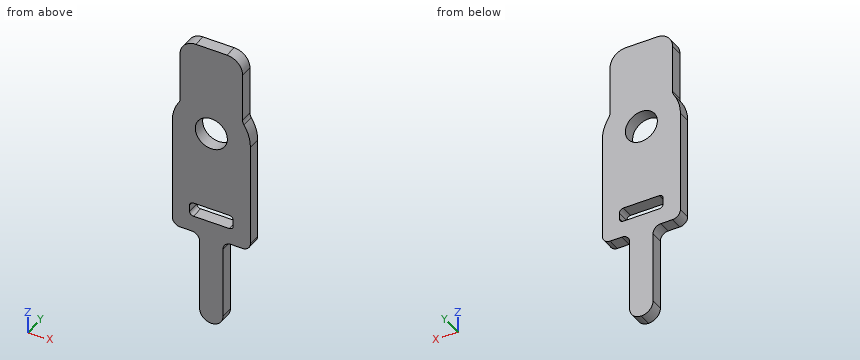
```python
from build123d import *

# Parameters (mm, degrees)
EXTRUDE_1_DEPTH = 1.6
FILLET_1_R      = 2
FILLET_2_R      = 1.5
FILLET_3_R      = 1
FILLET_4_R      = 0.5


with BuildPart() as part:
    # 草图1 → 凸台-拉伸1 (new body)
    with BuildSketch(Plane(origin=(0, 0, 0), x_dir=(1, 0, 0), z_dir=(0, 1, 0))):
        with BuildLine():
            Line((0, 37.4), (1.5, 37.4))
            Line((1.5, 37.4), (1.5, 25.7))
            Line((1.5, 25.7), (5, 25.7))
            Line((5, 25.7), (5, 11.5))
            ThreePointArc((5, 11.5), (4.74341649, 9.91886117), (4, 8.5))
            Line((4, 8.5), (4, 0))
            Line((4, 0), (0, 0))
            Line((0, 0), (0, 9.45))
            ThreePointArc((0, 9.45), (2.05, 11.5), (0, 13.55))
            Line((0, 13.55), (0, 21.8))
            Line((0, 21.8), (2.8, 21.8))
            Line((2.8, 21.8), (2.8, 23.6))
            Line((2.8, 23.6), (0, 23.6))
            Line((0, 23.6), (0, 37.4))
        make_face()
    extrude(amount=EXTRUDE_1_DEPTH)

    # 圆角1
    fillet_1_edges = [part.edges().sort_by_distance(p)[0] for p in [
        (4, 0.8, 0),
    ]]
    fillet(fillet_1_edges, radius=FILLET_1_R)

    # 圆角2
    fillet_2_edges = [part.edges().sort_by_distance(p)[0] for p in [
        (1.5, 0.8, -37.4),
    ]]
    fillet(fillet_2_edges, radius=FILLET_2_R - 0.0001)  # a hair under: the kernel refuses the full size

    # 圆角3
    fillet_3_edges = [part.edges().sort_by_distance(p)[0] for p in [
        (1.5, 0.8, -25.7),
        (5, 0.8, -25.7),
        (4, 0.8, -8.5),
    ]]
    fillet(fillet_3_edges, radius=FILLET_3_R)

    # 圆角4
    fillet_4_edges = [part.edges().sort_by_distance(p)[0] for p in [
        (2.8, 0.8, -21.8),
        (2.8, 0.8, -23.6),
    ]]
    fillet(fillet_4_edges, radius=FILLET_4_R)

    # 镜向1: part across plane


with BuildPart() as part_1:
    add(part.part)
    add(part.part.mirror(Plane(origin=(0, 1.6, -37.4), x_dir=(0, 0, 1), z_dir=(1, 0, 0))))


solid = part_1.part
```
The listing builds one solid part. Answer for the finished solid, in the listing's coordinates (mm). Give positions to 0.01 mm unless a question says otherwise; leave off trailing zeros. Order: outer loops, then holes, each group sorted by start corner. A loop starts at its lowest first (then second) coordinate and runs counter-clockwise, first axis right, second up. Notation, with made-up numbers: (30, 16.5) -> (42, 16.5) arc R10 cw to (42, 26.5) -> close; hole circle Ø8 at (12.25, 1). An arc over 180 degrees is marked (long way). Answer as CSV lines item,"result". Start each with the question number.
Q1. Find the intervals of material crossed by L1, parallel to Z at x = -0.75, y = 1.2; L2, parallel to X at y = 0.5, z = -11.5; L3, parallel to X at y = 0.9, z = -22.5, in increasing order.
Q2. Given pin 1 (0.5 mm diameter, centred on y = 1, z = -5, fed in from -X); pin 2 (2 mm diameter, centred on x = -0.5, z = -19.5, fed in from -Y); pin 3 (0.8 mm diameter, centred on y = 1, z = -30.5, fed in from +X), each flat-ended and moving along its own axis, determine where each tip first touches the part or whether it passes through.
Q3. A cutting plane is placed at A-A (y = 0.55). Count the separate pieces of the cut face and the enclosed holes in it, then the cut area to 3 significant figures.
Q4. A cutting plane is placed at D-D (z = -32). Determine the outline of the cut face in (x, y), then the cut area to 3 significant figures.
Q5. A cutting plane is placed at C-C (z = -10). Determine the outline of the cut face in (x, y).
Q6. A cutting plane is placed at B-B (x = 0.5). Determine the outline of the cut face in (y, z).
Results found:
1,L1,"-37.2 to -23.6, -21.8 to -13.41, -9.59 to 0"
1,L2,"-5 to -2.05, 2.05 to 5"
1,L3,"-5 to -2.8, 2.8 to 5"
2,pin 1,"x = -4"
2,pin 2,"y = 0"
2,pin 3,"x = 1.5"
3,separate pieces,"1"
3,enclosed holes,"2"
3,area,"247 mm2"
4,outline,"(-1.5, 0) -> (1.5, 0) -> (1.5, 1.6) -> (-1.5, 1.6) -> close"
4,area,"4.80 mm2"
5,outline,"(-4.77, 0) -> (-1.4, 0) -> (-1.4, 1.6) -> (-4.77, 1.6) -> close; (1.4, 0) -> (4.77, 0) -> (4.77, 1.6) -> (1.4, 1.6) -> close"
6,outline,"(0, -37.31) -> (1.6, -37.31) -> (1.6, -23.6) -> (0, -23.6) -> close; (0, -21.8) -> (1.6, -21.8) -> (1.6, -13.49) -> (0, -13.49) -> close; (0, -9.51) -> (1.6, -9.51) -> (1.6, 0) -> (0, 0) -> close"
